Geometry: final body of the model. Coordinates: model frame, mm. A direction names the side the tool comes from. Coordinates: 2 decimals unless noted, no trailing zeros. Order: outer loops, then holes, each group sorted by start corner. A loop starts at its lowest first (then second) coordinate and runs counter-clockwise, first axis right, second up. Notation, with made-up numbers: (4, -25) - (44, -25) arc R31 cw to (44, 13) - close; hole circle Ø10 at (24.5, 63). An arc over 180 degrees is marked (long way). Use one line per item in the form item = value. Start each with the question number.
```python
from build123d import *

# Parameters (mm, degrees)
EXTRUDE_1_DEPTH      = 15
EXTRUDE_1_DEPTH_BACK = 15
EXTRUDE_START        = -15
EXTRUDE_2_DEPTH      = 5
EXTRUDE_2_DEPTH_BACK = 5
SKETCH_3_R           = 1.5
CUT_EXTRUDE_1_DEPTH  = 11
SKETCH_4_R           = 1.5
CUT_EXTRUDE_2_DEPTH  = 11
CUT_EXTRUDE_3_DEPTH  = 1


with BuildPart() as part:
    # Sketch 1 → Extrude 1 (new body, two sides)
    with BuildSketch(Plane(origin=(0, 0, 0), x_dir=(0, 0, -1), z_dir=(1, 0, 0))) as extrude_1_sk:
        with BuildLine():
            Line((-40, -0.344795888), (-40, 36.655204112))
            ThreePointArc((-40, 36.655204112), (-39.121320344, 38.776524455), (-37, 39.655204112))
            Line((-37, 39.655204112), (37, 39.655204112))
            ThreePointArc((37, 39.655204112), (39.121320344, 38.776524455), (40, 36.655204112))
            Line((40, 36.655204112), (40, -0.344795888))
            Line((40, -0.344795888), (54, -0.344795888))
            Line((54, -0.344795888), (54, 2.655204112))
            Line((54, 2.655204112), (47, 2.655204112))
            ThreePointArc((47, 2.655204112), (44.878679656, 3.533883768), (44, 5.655204112))
            Line((44, 5.655204112), (44, 40.655204112))
            ThreePointArc((44, 40.655204112), (43.121320344, 42.776524455), (41, 43.655204112))
            Line((41, 43.655204112), (-41, 43.655204112))
            ThreePointArc((-41, 43.655204112), (-43.121320344, 42.776524455), (-44, 40.655204112))
            Line((-44, 40.655204112), (-44, 5.655204112))
            ThreePointArc((-44, 5.655204112), (-44.878679656, 3.533883768), (-47, 2.655204112))
            Line((-47, 2.655204112), (-54, 2.655204112))
            Line((-54, 2.655204112), (-54, -0.344795888))
            Line((-54, -0.344795888), (-40, -0.344795888))
        make_face()
    extrude(amount=EXTRUDE_1_DEPTH)
    extrude(extrude_1_sk.sketch, amount=-EXTRUDE_1_DEPTH_BACK)

    # Sketch 2 → Extrude 2 (add, two sides)
    with BuildSketch(Plane(origin=(15, 0, 0), x_dir=(0, 0, -1), z_dir=(1, 0, 0)).offset(EXTRUDE_START)) as extrude_2_sk:
        with BuildLine():
            Line((-52.25, 56.016603057), (-46, 56.016603057))
            Line((-46, 56.016603057), (-46, 52.016603057))
            Line((-46, 52.016603057), (-50.520133989, 52.016603057))
            ThreePointArc((-50.520133989, 52.016603057), (-51.385897915, 47.874388257), (-52.830611648, 43.896915082))
            Line((-52.830611648, 43.896915082), (-44, 40.655204112))
            Line((-44, 40.655204112), (-44, 23.155204112))
            Line((-44, 23.155204112), (-80, 26.266603057))
            ThreePointArc((-80, 26.266603057), (-99.571184175, 33.610549187), (-109.479866011, 52.016603057))
            Line((-109.479866011, 52.016603057), (-114, 52.016603057))
            Line((-114, 52.016603057), (-114, 56.016603057))
            Line((-114, 56.016603057), (-107.75, 56.016603057))
            ThreePointArc((-107.75, 56.016603057), (-80, 28.266603057), (-52.25, 56.016603057))
        make_face()
        with BuildLine():
            Line((52.830611648, 43.896915082), (44, 40.655204112))
            Line((44, 40.655204112), (44, 23.155204112))
            Line((44, 23.155204112), (80, 26.266603057))
            ThreePointArc((80, 26.266603057), (99.571184175, 33.610549187), (109.479866011, 52.016603057))
            Line((109.479866011, 52.016603057), (114, 52.016603057))
            Line((114, 52.016603057), (114, 56.016603057))
            Line((114, 56.016603057), (107.75, 56.016603057))
            ThreePointArc((107.75, 56.016603057), (80, 28.266603057), (52.25, 56.016603057))
            Line((52.25, 56.016603057), (46, 56.016603057))
            Line((46, 56.016603057), (46, 52.016603057))
            Line((46, 52.016603057), (50.520133989, 52.016603057))
            ThreePointArc((50.520133989, 52.016603057), (51.385897915, 47.874388257), (52.830611648, 43.896915082))
        make_face()
    extrude(amount=EXTRUDE_2_DEPTH)
    extrude(extrude_2_sk.sketch, amount=-EXTRUDE_2_DEPTH_BACK)

    # Sketch 3 → Cut-Extrude 1 (cut)
    with BuildSketch(Plane(origin=(0, 56.016603057, 0), x_dir=(1, 0, 0), z_dir=(0, 1, 0))):
        with Locations((0, 109.7)):
            Circle(SKETCH_3_R)
        with Locations((0, 50.3)):
            Circle(SKETCH_3_R)
        with Locations((0, -50.3)):
            Circle(SKETCH_3_R)
        with Locations((0, -109.7)):
            Circle(SKETCH_3_R)
    extrude(amount=-CUT_EXTRUDE_1_DEPTH, mode=Mode.SUBTRACT)

    # Sketch 4 → Cut-Extrude 2 (cut)
    with BuildSketch(Plane(origin=(0, 2.655204112, 0), x_dir=(1, 0, 0), z_dir=(0, 1, 0))):
        with Locations((-12, -51)):
            Circle(SKETCH_4_R)
        with Locations((12, -51)):
            Circle(SKETCH_4_R)
        with Locations((12, 51)):
            Circle(SKETCH_4_R)
        with Locations((-12, 51)):
            Circle(SKETCH_4_R)
    extrude(amount=-CUT_EXTRUDE_2_DEPTH, mode=Mode.SUBTRACT)

    # Sketch 5 → Cut-Extrude 3 (cut)
    with BuildSketch(Plane(origin=(0, 2.655204112, 0), x_dir=(1, 0, 0), z_dir=(0, 1, 0))):
        Polygon((-12, 54.175426481), (-14.75, 52.58771324), (-14.75, 49.41228676), (-12, 47.824573519), (-9.25, 49.41228676), (-9.25, 52.58771324), align=None)
        Polygon((12, 54.175426481), (9.25, 52.58771324), (9.25, 49.41228676), (12, 47.824573519), (14.75, 49.41228676), (14.75, 52.58771324), align=None)
        Polygon((14.75, -52.58771324), (12, -54.175426481), (9.25, -52.58771324), (9.25, -49.41228676), (12, -47.824573519), (14.75, -49.41228676), align=None)
        Polygon((-9.25, -52.58771324), (-12, -54.175426481), (-14.75, -52.58771324), (-14.75, -49.41228676), (-12, -47.824573519), (-9.25, -49.41228676), align=None)
    extrude(amount=-CUT_EXTRUDE_3_DEPTH, mode=Mode.SUBTRACT)


solid = part.part
```
(1) Cut plane C-C on z = 13.5. Return the cut outline in (x, y), plus the area to 3 significant figures.
(2) Contact query for flat-ended pins moving along their axis: pin 1 Ø7.5 at (x, z) = (-6, -52) entering from +Y; pin 2 Ø6 at (x, z) = (-11, -51.5) entering from +Y; pin 3 Ø1.5 at (x, y) = (-1.5, 0.5) entering from +Z; pin 4 Ø4 at (x, z) = (-12, 51) entering from +Y. Output: stop coordinate, or through.
(3) Draft query along Z for faces 5 (the flat face through (0, 54, -114)), 6 (the flat face through (0, 43.655, -1)), 7 (the flat face through (0, 54, 114)), 8 (the flat face through (0, 56.017, 112)). Return one class per face: released by +Z, released by -Z, zero draft, split by the parting line, or undercut.
(4) Cut plane B-B on y = 31.5. Return the cut outline in (x, z).
(5) Material intervals for L1, parallel to Z at x = 12, y = 1.2; L2, parallel to X at y = 1, z = 51; L3, parallel to Z at x = 0.25, y = 51, sorted ascending. Write a range as from..to.
(6) Set-up query: faces 1 (the flat face through (0, 23, -44)), 2 (the flat face through (-5, 32, 63)), 3 (the flat face through (0, 20, 44)), 4 (the flat face through (5, 32, -63)). Return all of +Z, -Z, +X, -X, +Y, -Y with unobstructed straight access to the full face (end or side cutting, diameter ignored); none if empty.
(7) Cut plane A-A on y = 8. Return the cut outline in (x, z), plus the area to 3 significant figures.
(8) Cut plane D-D on z = -59.5. Return the cut outline in (x, y).
Check sheet entries:
q1.outline = (-15, 39.66) - (15, 39.66) - (15, 43.66) - (-15, 43.66) - close
q1.area = 120 mm^2
q2.pin_1 = 56.02
q2.pin_2 = 2.66
q2.pin_3 = 54
q2.pin_4 = 1.66
q3.face_5 = released by -Z
q3.face_6 = undercut
q3.face_7 = released by +Z
q3.face_8 = zero draft
q4.outline = (-15, -44) - (-5, -44) - (-5, -67) - (5, -67) - (5, -44) - (15, -44) - (15, -40) - (-15, -40) - close; (-15, 40) - (15, 40) - (15, 44) - (5, 44) - (5, 67) - (-5, 67) - (-5, 44) - (-15, 44) - close; (-5, -96.85) - (5, -96.85) - (5, -93) - (-5, -93) - close; (-5, 93) - (5, 93) - (5, 96.85) - (-5, 96.85) - close
q5.L1 = -54..-52.5, -49.5..-40, 40..49.5, 52.5..54
q5.L2 = -15..-13.5, -10.5..10.5, 13.5..15
q5.L3 = -108.22..-107.29, -52.71..-51.78, 51.78..52.71, 107.29..108.22
q6.face_1 = -Z
q6.face_2 = +Z, -X, +Y
q6.face_3 = +Z
q6.face_4 = -Z, +X, +Y
q7.outline = (-15, -44) - (15, -44) - (15, -40) - (-15, -40) - close; (-15, 40) - (15, 40) - (15, 44) - (-15, 44) - close
q7.area = 240 mm^2
q8.outline = (-5, 24.49) - (5, 24.49) - (5, 37.31) - (-5, 37.31) - close
